```python
from build123d import *

# Parameters (mm, degrees)
F0_W         = 200
F0_H         = 130
F0_W_2       = 0.3
F0_H_2       = 106.96
F1_DEPTH     = 2
F2_DEPTH     = 14
F3_DEPTH     = 8
F4_D         = 2
F5_R         = 5
F6_T         = 2
F6_T3_DEPTH  = 16
F6_T5_DEPTH  = 10
F6_T7_DEPTH  = 12
F6_T9_DEPTH  = 10
F6_T11_DEPTH = 153.2
F6_T13_DEPTH = 12
F6_T15_DEPTH = 4.3
F6_T17_DEPTH = 129
F6_T19_DEPTH = 12.3
F6_T21_DEPTH = 11.7
F6_T23_DEPTH = 153.2
F6_T25_DEPTH = 13.02
F6_T27_DEPTH = 13.02
F6_T29_DEPTH = 110.96
F7_W         = 23
F7_H         = 2
F8_DEPTH     = 22.5
F9_W         = 50
F9_H         = 8
F9_H_2       = 2
F10_DEPTH    = 25


# Not quite as in the source:
# - a shell that OpenCascade refuses in one call is made with other operations: the cavity is built on its own and cut out


with BuildPart() as f1:
    # F0 (on Top) → F1 (new body)
    with BuildSketch(Plane.XY):
        Rectangle(F0_W, F0_H)
        Polygon((77.15, 62.5), (79.15, 62.5), (82.45, 62.5), (82.75, 62.5), (82.75, 59.5), (82.75, -58.77), (82.75, -62.5), (82.45, -62.5), (79.45, -62.5), (77.45, -62.5), (74.75, -62.5), (-74.45, -62.5), (-77.45, -62.5), (-79.45, -62.5), (-82.75, -62.5), (-82.75, -58.77), (-82.75, -53.48), (-82.75, 53.48), (-82.75, 59.5), (-82.75, 62.5), (-79.75, 62.5), (-77.75, 62.5), (-74.75, 62.5), (74.45, 62.5), align=None, mode=Mode.SUBTRACT)
        Polygon((74.45, 53.48), (74.45, 62.5), (-74.75, 62.5), (-74.75, 53.48), (-82.45, 53.48), (-82.45, -53.48), (-74.45, -53.48), (-74.45, -62.5), (74.75, -62.5), (74.75, -53.48), (82.45, -53.48), (82.45, 53.48), align=None)
        Polygon((-74.75, 53.48), (-74.75, 62.5), (-77.75, 62.5), (-79.75, 62.5), (-82.75, 62.5), (-82.75, 59.5), (-82.75, 53.48), (-82.45, 53.48), align=None)
        Polygon((82.45, 62.5), (79.15, 62.5), (77.15, 62.5), (74.45, 62.5), (74.45, 53.48), (82.45, 53.48), align=None)
        Polygon((82.45, -62.5), (82.45, -53.48), (74.75, -53.48), (74.75, -62.5), (77.45, -62.5), (79.45, -62.5), align=None)
        Polygon((-74.45, -53.48), (-82.45, -53.48), (-82.75, -53.48), (-82.75, -58.77), (-82.75, -62.5), (-79.45, -62.5), (-77.45, -62.5), (-74.45, -62.5), align=None)
        with Locations((-82.6, 0)):
            Rectangle(F0_W_2, F0_H_2)
        Polygon((82.75, 62.5), (82.45, 62.5), (82.45, 53.48), (82.45, -53.48), (82.45, -62.5), (82.75, -62.5), (82.75, -58.77), (82.75, 59.5), align=None)
    extrude(amount=F1_DEPTH)

    # F0 (on Top) → F2 (join)
    with BuildSketch(Plane.XY):
        Rectangle(F0_W, F0_H)
        Polygon((77.15, 62.5), (79.15, 62.5), (82.45, 62.5), (82.75, 62.5), (82.75, 59.5), (82.75, -58.77), (82.75, -62.5), (82.45, -62.5), (79.45, -62.5), (77.45, -62.5), (74.75, -62.5), (-74.45, -62.5), (-77.45, -62.5), (-79.45, -62.5), (-82.75, -62.5), (-82.75, -58.77), (-82.75, -53.48), (-82.75, 53.48), (-82.75, 59.5), (-82.75, 62.5), (-79.75, 62.5), (-77.75, 62.5), (-74.75, 62.5), (74.45, 62.5), align=None, mode=Mode.SUBTRACT)
    extrude(amount=F2_DEPTH)

    # F0 (on Top) → F3 (join)
    with BuildSketch(Plane.XY):
        Polygon((-74.45, -53.48), (-82.45, -53.48), (-82.75, -53.48), (-82.75, -58.77), (-82.75, -62.5), (-79.45, -62.5), (-77.45, -62.5), (-74.45, -62.5), align=None)
        Polygon((-74.75, 53.48), (-74.75, 62.5), (-77.75, 62.5), (-79.75, 62.5), (-82.75, 62.5), (-82.75, 59.5), (-82.75, 53.48), (-82.45, 53.48), align=None)
        Polygon((82.45, -62.5), (82.45, -53.48), (74.75, -53.48), (74.75, -62.5), (77.45, -62.5), (79.45, -62.5), align=None)
        Polygon((82.45, 62.5), (79.15, 62.5), (77.15, 62.5), (74.45, 62.5), (74.45, 53.48), (82.45, 53.48), align=None)
    extrude(amount=F3_DEPTH)

    # F4 (through all)
    with Locations(Plane(origin=(0, 0, 0), x_dir=(1, 0, 0), z_dir=(0, 0, -1))):
        with Locations((-78.45, 57.48), (78.45, 57.48), (-78.45, -57.48), (78.45, -57.48)):
            Hole(F4_D / 2)

    # F5
    f5_edges = [f1.edges().sort_by_distance(p)[0] for p in [
        (-100, -65, 7),
        (-100, 65, 7),
        (100, 65, 7),
        (100, -65, 7),
    ]]
    fillet(f5_edges, radius=F5_R)

    # F6: shell of thickness 2, made by hand


with BuildPart() as f6_core1:
    # F6_t2: copy of F1
    add(f1.part)

    # the walls: a layer under each face that stays
    f6_faces = [f6_core1.faces().sort_by_distance(p)[0] for p in [
        (100, 0, 7),
        (98.5355339059, -63.5355339059, 7),
        (98.5355339059, 63.5355339059, 7),
        (0, 0, 0),
        (0, -65, 7),
        (0, 65, 7),
        (-98.5355339059, -63.5355339059, 7),
        (-98.5355339059, 63.5355339059, 7),
        (-100, 0, 7),
        (0, 62.5, 8),
        (82.75, 0, 8),
        (0, -62.5, 8),
        (-82.75, 0, 8),
        (-79.45, -57.48, 4),
        (77.45, -57.48, 4),
        (-79.45, 57.48, 4),
        (77.45, 57.48, 4),
        (-81.4166666667, 54.9833333333, 8),
        (-74.75, 57.99, 5),
        (0, 0, 2),
        (74.45, 57.99, 5),
        (75.7833333333, 54.9833333333, 8),
        (82.45, 57.99, 5),
        (-74.45, -57.99, 5),
        (-81.3666666667, -60.9966666667, 8),
        (82.45, -57.99, 5),
        (76.0333333333, -60.9966666667, 8),
        (74.75, -57.99, 5),
        (-78.75, 53.48, 5),
        (-78.6, -53.48, 5),
        (78.6, -53.48, 5),
        (78.45, 53.48, 5),
    ]]
    thicken(f6_faces, amount=-F6_T, mode=Mode.SUBTRACT)

    # F6_s4 → F6_t3 (cut)
    with BuildSketch(Plane.XY):
        Polygon((82.73, 62.48), (82.75, 64.5), (84.75, 64.5), (84.75, 62.5), align=None)
        Polygon((82.73, -62.48), (84.75, -62.5), (84.75, -64.5), (82.75, -64.5), align=None)
    extrude(amount=F6_T3_DEPTH, mode=Mode.SUBTRACT)

    # F6_s6 → F6_t5 (cut)
    with BuildSketch(Plane.XY.offset(6)):
        Polygon((-82.73, 62.48), (-82.75, 64.5), (-84.75, 64.5), (-84.75, 62.5), align=None)
        Polygon((-82.73, -62.48), (-82.75, -64.5), (-84.75, -64.5), (-84.75, -62.5), align=None)
    extrude(amount=F6_T5_DEPTH, mode=Mode.SUBTRACT)

    # F6_s8 → F6_t7 (cut)
    with BuildSketch(Plane.YZ.offset(-84.75)):
        Polygon((62.48, 8.02), (64.5, 8), (64.5, 6), (62.5, 6), align=None)
        Polygon((53.46, 2.02), (53.48, 0), (55.48, 0), (55.48, 2), align=None)
    extrude(amount=F6_T7_DEPTH, mode=Mode.SUBTRACT)

    # F6_s10 → F6_t9 (cut)
    with BuildSketch(Plane.XY):
        Polygon((-74.73, 62.48), (-74.75, 64.5), (-76.75, 64.5), (-76.75, 62.5), align=None)
        Polygon((74.43, 62.48), (74.45, 64.5), (76.45, 64.5), (76.45, 62.5), align=None)
        Polygon((82.47, 62.48), (82.45, 64.5), (80.45, 64.5), (80.45, 62.5), align=None)
        Polygon((-74.43, -62.48), (-74.45, -64.5), (-76.45, -64.5), (-76.45, -62.5), align=None)
        Polygon((82.47, -62.48), (82.45, -64.5), (80.45, -64.5), (80.45, -62.5), align=None)
        Polygon((74.73, -62.48), (74.75, -64.5), (76.75, -64.5), (76.75, -62.5), align=None)
        Polygon((-82.73, 53.46), (-84.75, 53.48), (-84.75, 55.48), (-82.75, 55.48), align=None)
        Polygon((-82.73, -53.46), (-84.75, -53.48), (-84.75, -55.48), (-82.75, -55.48), align=None)
    extrude(amount=F6_T9_DEPTH, mode=Mode.SUBTRACT)

    # F6_s12 → F6_t11 (cut)
    with BuildSketch(Plane.YZ.offset(-76.75)):
        Polygon((62.48, 2.02), (64.5, 2), (64.5, 0), (62.5, 0), align=None)
    extrude(amount=F6_T11_DEPTH, mode=Mode.SUBTRACT)

    # F6_s14 → F6_t13 (cut)
    with BuildSketch(Plane.YZ.offset(72.45)):
        Polygon((62.48, 8.02), (64.5, 8), (64.5, 6), (62.5, 6), align=None)
        Polygon((53.46, 2.02), (53.48, 0), (55.48, 0), (55.48, 2), align=None)
    extrude(amount=F6_T13_DEPTH, mode=Mode.SUBTRACT)

    # F6_s16 → F6_t15 (cut)
    with BuildSketch(Plane.YZ.offset(80.45)):
        Polygon((62.48, 2.02), (64.5, 2), (64.5, 0), (62.5, 0), align=None)
        Polygon((-62.48, 2.02), (-64.5, 2), (-64.5, 0), (-62.5, 0), align=None)
    extrude(amount=F6_T15_DEPTH, mode=Mode.SUBTRACT)

    # F6_s18 → F6_t17 (cut)
    with BuildSketch(Plane.XZ.offset(-64.5)):
        Polygon((82.73, 2.02), (84.75, 2), (84.75, 0), (82.75, 0), align=None)
    extrude(amount=F6_T17_DEPTH, mode=Mode.SUBTRACT)

    # F6_s20 → F6_t19 (cut)
    with BuildSketch(Plane.YZ.offset(-84.75)):
        Polygon((-62.48, 8.02), (-64.5, 8), (-64.5, 6), (-62.5, 6), align=None)
        Polygon((-53.46, 2.02), (-53.48, 0), (-55.48, 0), (-55.48, 2), align=None)
    extrude(amount=F6_T19_DEPTH, mode=Mode.SUBTRACT)

    # F6_s22 → F6_t21 (cut)
    with BuildSketch(Plane.YZ.offset(72.75)):
        Polygon((-62.48, 8.02), (-64.5, 8), (-64.5, 6), (-62.5, 6), align=None)
        Polygon((-53.46, 2.02), (-53.48, 0), (-55.48, 0), (-55.48, 2), align=None)
    extrude(amount=F6_T21_DEPTH, mode=Mode.SUBTRACT)

    # F6_s24 → F6_t23 (cut)
    with BuildSketch(Plane.YZ.offset(-76.45)):
        Polygon((-62.48, 2.02), (-64.5, 2), (-64.5, 0), (-62.5, 0), align=None)
    extrude(amount=F6_T23_DEPTH, mode=Mode.SUBTRACT)

    # F6_s26 → F6_t25 (cut)
    with BuildSketch(Plane.XZ.offset(-64.5)):
        Polygon((-82.73, 8.02), (-84.75, 8), (-84.75, 6), (-82.75, 6), align=None)
        Polygon((-74.73, 2.02), (-76.75, 2), (-76.75, 0), (-74.75, 0), align=None)
        Polygon((74.43, 2.02), (74.45, 0), (76.45, 0), (76.45, 2), align=None)
        Polygon((82.47, 2.02), (82.45, 0), (80.45, 0), (80.45, 2), align=None)
    extrude(amount=F6_T25_DEPTH, mode=Mode.SUBTRACT)

    # F6_s28 → F6_t27 (cut)
    with BuildSketch(Plane.XZ.offset(51.48)):
        Polygon((-82.73, 8.02), (-84.75, 8), (-84.75, 6), (-82.75, 6), align=None)
        Polygon((82.47, 2.02), (82.45, 0), (80.45, 0), (80.45, 2), align=None)
        Polygon((74.73, 2.02), (74.75, 0), (76.75, 0), (76.75, 2), align=None)
        Polygon((-74.43, 2.02), (-74.45, 0), (-76.45, 0), (-76.45, 2), align=None)
    extrude(amount=F6_T27_DEPTH, mode=Mode.SUBTRACT)

    # F6_s30 → F6_t29 (cut)
    with BuildSketch(Plane.XZ.offset(-55.48)):
        Polygon((-82.73, 2.02), (-84.75, 2), (-84.75, 0), (-82.75, 0), align=None)
    extrude(amount=F6_T29_DEPTH, mode=Mode.SUBTRACT)


with BuildPart() as f1_1:
    add(f1.part)

    # what is left inside the walls is the cavity
    f6_cavity = [f6_core1.part.solids().sort_by_distance(p)[0] for p in [
        (91.375, -21, 13.98),
        (-87.225, -21, 2.02),
        (78.642053, -60.493887, 4.666667),
        (78.45, 60.5, 4.666667),
    ]]
    add(f6_cavity, mode=Mode.SUBTRACT)

    # F7 (on face) → F8 (cut)
    with BuildSketch(Plane(origin=(0, 0, 0), x_dir=(1, 0, 0), z_dir=(0, 0, -1))):
        with Locations((-68.5, 49)):
            Rectangle(F7_W, F7_H)
        with Locations((-68.5, 37)):
            Rectangle(F7_W, F7_H)
        with Locations((-68.5, -37)):
            Rectangle(F7_W, F7_H)
        with Locations((-68.5, -49)):
            Rectangle(F7_W, F7_H)
    extrude(amount=-F8_DEPTH, mode=Mode.SUBTRACT)

    # F9 (on face) → F10 (cut)
    with BuildSketch(Plane.YZ.offset(-82.75)):
        with Locations((0, 8)):
            Rectangle(F9_W, F9_H)
        with Locations((0, 13)):
            Rectangle(F9_W, F9_H_2)
    extrude(amount=-F10_DEPTH, mode=Mode.SUBTRACT)


solid = f1_1.part
```
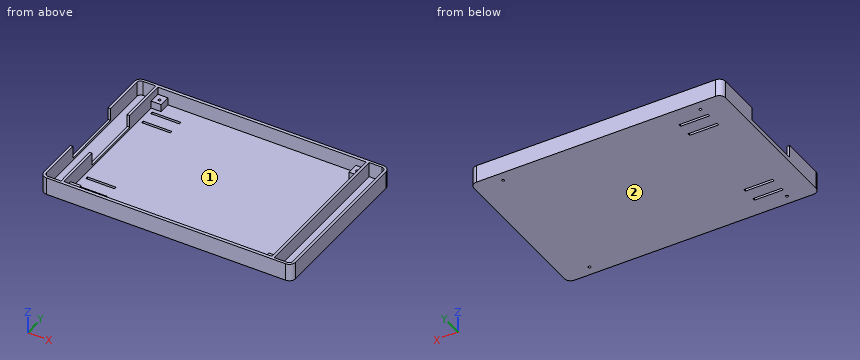
Here's how the part is built. I have some questions about the finished solid (model axes, mm). Face numbers are marked on the shaded views. Round coordinates to 2 decimals unless told otherwise and drop trailing zeros. Loops run counter-clockwise (first coordinate to the right, second up) from the corner with the lowest first, then second, coordinate; pieces in that order, holes last. Notation, with made-up numbers: (12.5, 87.25) -> (26.5, 87.25) arc R27 cw to (26.5, 107.25) -> close; hole circle Ø10 at (79.25, 72). An arc over 180 degrees is marked (long way). Answer as CSV lines item,"result". Start each with the question number.
1. I need wall thicknesses on probe 1 along X at (y, z) = (-30, 3); probe 2 along Y at (x, z) = (78.45, 5); probe 3 along Y at (x, z) = (-42.5, 12.25). Which ranges of each line are inside material? Lowest first, please. Write a range as from..to.
2. Imagine slicing it at C-C on x = 2. Write out the boundary of the cut face in (y, z), plus the area to 3 significant figures.
3. Imagine slicing it at B-B on y = 14.5. Write out the boundary of the cut face in (x, z), plus the area to 3 significant figures.
4. If we mould it in two halves opening along Y, with no side actions, what happens to the marked faces 1 and 2? For each: pulls with the +Y half, pulls with the -Y half, needs draft (parallel to the pull), parting line crosses it, or undercut.
5. I'm going to push flat-ended pins straight in: P1, Ø1.6, axis at x = 78.45, y = 57.48, coming from the +Z side; P2, Ø6, axis at y = 21.5, z = 10.5, coming from the -X side; P3, Ø4, axis at x = -79, y = -57, coming from the +Z side; P4, Ø2.5, axis at y = -62, z = 5, coming from the +X side. Where does each tip first touch, or does it pass through?
Solution:
1,probe 1,"-100..-98, -84.75..-82.75, 82.75..84.75, 98..100"
1,probe 2,"-65..-63, -60.48..-58.48, -56.48..-53.48, 53.48..56.48, 58.48..60.48, 63..65"
1,probe 3,"-65..-62.5, 62.5..65"
2,outline,"(-65, 0) -> (65, 0) -> (65, 14) -> (62.5, 14) -> (62.5, 2) -> (-62.5, 2) -> (-62.5, 14) -> (-65, 14) -> close"
2,area,"320 mm²"
3,outline,"(-100, 0) -> (100, 0) -> (100, 14) -> (98, 14) -> (98, 2) -> (84.75, 2) -> (84.75, 14) -> (82.75, 14) -> (82.75, 2) -> (-82.75, 2) -> (-82.75, 4) -> (-84.75, 4) -> (-84.75, 2) -> (-98, 2) -> (-98, 4) -> (-100, 4) -> close"
3,area,"456 mm²"
4,face 1,"undercut"
4,face 2,"needs draft"
5,P1,"through"
5,P2,"x = 82.75"
5,P3,"z = 8"
5,P4,"x = 99.94"
